Input: part model. Units: mm. Frame: model coordinates. Give positions to 0.01 mm unless a question says otherwise; leave off trailing zeros. Loops run counter-clockwise (first coordinate to the right, second up) from the corner with the lowest first, then second, coordinate; pieces in that order, holes last. Notation, with made-up numbers: M 12.5,71.25 L 45.5,71.25 A32 ccw 45.5,105.25 Z; hole C 13.25,24.25 d11. An arc over 180 degrees is marked long. Return JSON: item names as keys, results as strings. Group by question number.
```python
from build123d import *

# Parameters (mm, degrees)
F0_W         = 57.15
F0_H         = 69.85
F1_DEPTH     = 25.4
F2_R         = 3.556
F3_DEPTH     = 25.4
F4_T1_DEPTH  = 82.55
F5_T1_DEPTH  = 77.47
F5_T3_DEPTH  = 33.02
F5_T6_ANGLE  = 89.9999999979
F6_T1_DEPTH  = 64.77
F6_T3_DEPTH  = 33.02
F6_T6_ANGLE  = 89.9999999979
F7_T1_DEPTH  = 59.69
F7_T3_DEPTH  = 33.02
F7_T6_ANGLE  = 89.9999999979
F7_T8_ANGLE  = 89.9999999979
F8_T1_DEPTH  = 59.69
F8_T3_DEPTH  = 46.99
F8_T6_ANGLE  = 89.9999999979
F8_T8_ANGLE  = 90.0000000017
F8_T10_ANGLE = 90.0000000017
F8_T12_ANGLE = 89.9999999979


# Not quite as in the source:
# - a fillet or chamfer that OpenCascade refuses, or shapes differently, is made with other operations: its cross-section is extruded or revolved along the edge and cut away or added


with BuildPart() as f1:
    # F0 (on Top) → F1 (new body)
    with BuildSketch(Plane.XY):
        with Locations((-11.2585859209, 15.0406121326)):
            Rectangle(F0_W, F0_H)
    extrude(amount=F1_DEPTH)

    # F2 (on face) → F3 (cut)
    with BuildSketch(Plane.XY.offset(25.4)):
        with Locations((-30.9435859209, 42.3456121326)):
            Circle(F2_R)
        with Locations((8.4264140791, 42.3456121326)):
            Circle(F2_R)
        with Locations((-30.9435859209, -12.2643878674)):
            Circle(F2_R)
        with Locations((8.4264140791, -12.2643878674)):
            Circle(F2_R)
    extrude(amount=-F3_DEPTH, mode=Mode.SUBTRACT)

    # F4: fillet of radius 5.08 on 1 edges, made by hand

    # F4_s2 → F4_t1 (cut)
    with BuildSketch(Plane.YZ.offset(-52.5335859209)):
        with BuildLine():
            ThreePointArc((-14.8043878674, 25.4), (-18.3964903158, 23.9121024484), (-19.8843878674, 20.32))
            Line((-19.8843878674, 20.32), (-19.8843878674, 25.4))
            Line((-19.8843878674, 25.4), (-14.8043878674, 25.4))
        make_face()
    extrude(amount=F4_T1_DEPTH, mode=Mode.SUBTRACT)

    # F5: fillet of radius 5.08 on 1 edges, made by hand

    # F5_s2 → F5_t1 (cut)
    with BuildSketch(Plane.XZ.offset(-62.6656121326)):
        with BuildLine():
            ThreePointArc((17.3164140791, 20.32), (15.8285165275, 23.9121024484), (12.2364140791, 25.4))
            Line((12.2364140791, 25.4), (17.3164140791, 25.4))
            Line((17.3164140791, 25.4), (17.3164140791, 20.32))
        make_face()
    extrude(amount=F5_T1_DEPTH, mode=Mode.SUBTRACT)

    # F5_s4 → F5_t3 (cut)
    with BuildSketch(Plane.XY.offset(-12.7)):
        with BuildLine():
            ThreePointArc((17.3164140791, -14.8043878674), (15.8285165275, -18.3964903158), (12.2364140791, -19.8843878674))
            Line((12.2364140791, -19.8843878674), (17.3164140791, -19.8843878674))
            Line((17.3164140791, -19.8843878674), (17.3164140791, -14.8043878674))
        make_face()
    extrude(amount=F5_T3_DEPTH, mode=Mode.SUBTRACT)

    # F5_s5 → F5_t6 (revolve, cut)
    with BuildSketch(Plane.XY.offset(20.3199999999)):
        with BuildLine():
            ThreePointArc((17.3164140791, -14.8043878674), (15.8285165275, -18.3964903158), (12.2364140791, -19.8843878674))
            Line((12.2364140791, -19.8843878674), (17.3164140791, -19.8843878674))
            Line((17.3164140791, -19.8843878674), (17.3164140791, -14.8043878674))
        make_face()
    revolve(axis=Axis((17.3164140791, -14.8043878673, 20.3199999999), (-1, 0, 0)), revolution_arc=F5_T6_ANGLE, mode=Mode.SUBTRACT)

    # F6: fillet of radius 5.08 on 1 edges, made by hand

    # F6_s2 → F6_t1 (cut)
    with BuildSketch(Plane.YZ.offset(-52.5335859209)):
        with BuildLine():
            ThreePointArc((49.9656121326, 20.32), (48.477714581, 23.9121024484), (44.8856121326, 25.4))
            Line((44.8856121326, 25.4), (49.9656121326, 25.4))
            Line((49.9656121326, 25.4), (49.9656121326, 20.32))
        make_face()
    extrude(amount=F6_T1_DEPTH, mode=Mode.SUBTRACT)

    # F6_s4 → F6_t3 (cut)
    with BuildSketch(Plane.XY.offset(-12.7)):
        with BuildLine():
            ThreePointArc((12.2364140791, 49.9656121326), (15.8285165275, 48.477714581), (17.3164140791, 44.8856121326))
            Line((17.3164140791, 44.8856121326), (17.3164140791, 49.9656121326))
            Line((17.3164140791, 49.9656121326), (12.2364140791, 49.9656121326))
        make_face()
    extrude(amount=F6_T3_DEPTH, mode=Mode.SUBTRACT)

    # F6_s5 → F6_t6 (revolve, cut)
    with BuildSketch(Plane.YZ.offset(12.236414079)):
        with BuildLine():
            ThreePointArc((49.9656121326, 20.32), (48.477714581, 23.9121024484), (44.8856121326, 25.4))
            Line((44.8856121326, 25.4), (49.9656121326, 25.4))
            Line((49.9656121326, 25.4), (49.9656121326, 20.32))
        make_face()
    revolve(axis=Axis((12.236414079, 49.9656121326, 20.3199999999), (0, 1, 0)), revolution_arc=F6_T6_ANGLE, mode=Mode.SUBTRACT)

    # F7: fillet of radius 5.08 on 1 edges, made by hand

    # F7_s2 → F7_t1 (cut)
    with BuildSketch(Plane.XZ.offset(-44.8856121326)):
        with BuildLine():
            ThreePointArc((-39.8335859209, 20.32), (-38.3456883694, 23.9121024484), (-34.7535859209, 25.4))
            Line((-34.7535859209, 25.4), (-39.8335859209, 25.4))
            Line((-39.8335859209, 25.4), (-39.8335859209, 20.32))
        make_face()
    extrude(amount=F7_T1_DEPTH, mode=Mode.SUBTRACT)

    # F7_s4 → F7_t3 (cut)
    with BuildSketch(Plane.XY.offset(-12.7)):
        with BuildLine():
            ThreePointArc((-39.8335859209, -14.8043878674), (-38.3456883694, -18.3964903158), (-34.7535859209, -19.8843878674))
            Line((-34.7535859209, -19.8843878674), (-39.8335859209, -19.8843878674))
            Line((-39.8335859209, -19.8843878674), (-39.8335859209, -14.8043878674))
        make_face()
        with BuildLine():
            ThreePointArc((-34.7535859209, 49.9656121326), (-38.3456883694, 48.477714581), (-39.8335859209, 44.8856121326))
            Line((-39.8335859209, 44.8856121326), (-39.8335859209, 49.9656121326))
            Line((-39.8335859209, 49.9656121326), (-34.7535859209, 49.9656121326))
        make_face()
    extrude(amount=F7_T3_DEPTH, mode=Mode.SUBTRACT)

    # F7_s5 → F7_t6 (revolve, cut)
    with BuildSketch(Plane.XZ.offset(-44.8856121325)):
        with BuildLine():
            ThreePointArc((-39.8335859209, 20.32), (-38.3456883694, 23.9121024484), (-34.7535859209, 25.4))
            Line((-34.7535859209, 25.4), (-39.8335859209, 25.4))
            Line((-39.8335859209, 25.4), (-39.8335859209, 20.32))
        make_face()
    revolve(axis=Axis((-39.8335859209, 44.8856121325, 20.3199999999), (-1, 0, 0)), revolution_arc=F7_T6_ANGLE, mode=Mode.SUBTRACT)

    # F7_s7 → F7_t8 (revolve, cut)
    with BuildSketch(Plane.XY.offset(20.3199999999)):
        with BuildLine():
            ThreePointArc((-39.8335859209, -14.8043878674), (-38.3456883694, -18.3964903158), (-34.7535859209, -19.8843878674))
            Line((-34.7535859209, -19.8843878674), (-39.8335859209, -19.8843878674))
            Line((-39.8335859209, -19.8843878674), (-39.8335859209, -14.8043878674))
        make_face()
    revolve(axis=Axis((-39.8335859209, -14.8043878673, 20.3199999999), (-1, 0, 0)), revolution_arc=F7_T8_ANGLE, mode=Mode.SUBTRACT)

    # F8: fillet of radius 5.08 on 8 edges, made by hand

    # F8_s2 → F8_t1 (cut)
    with BuildSketch(Plane.XZ.offset(-44.8856121326)):
        with BuildLine():
            ThreePointArc((-34.7535859209, 0), (-38.3456883694, 1.4878975516), (-39.8335859209, 5.08))
            Line((-39.8335859209, 5.08), (-39.8335859209, 0))
            Line((-39.8335859209, 0), (-34.7535859209, 0))
        make_face()
        with BuildLine():
            ThreePointArc((12.2364140791, 0), (15.8285165275, 1.4878975516), (17.3164140791, 5.08))
            Line((17.3164140791, 5.08), (17.3164140791, 0))
            Line((17.3164140791, 0), (12.2364140791, 0))
        make_face()
    extrude(amount=F8_T1_DEPTH, mode=Mode.SUBTRACT)

    # F8_s4 → F8_t3 (cut)
    with BuildSketch(Plane.YZ.offset(-34.7535859209)):
        with BuildLine():
            ThreePointArc((49.9656121326, 5.08), (48.477714581, 1.4878975516), (44.8856121326, 0))
            Line((44.8856121326, 0), (49.9656121326, 0))
            Line((49.9656121326, 0), (49.9656121326, 5.08))
        make_face()
        with BuildLine():
            ThreePointArc((-14.8043878674, 0), (-18.3964903158, 1.4878975516), (-19.8843878674, 5.08))
            Line((-19.8843878674, 5.08), (-19.8843878674, 0))
            Line((-19.8843878674, 0), (-14.8043878674, 0))
        make_face()
    extrude(amount=F8_T3_DEPTH, mode=Mode.SUBTRACT)

    # F8_s5 → F8_t6 (revolve, cut)
    with BuildSketch(Plane.XZ.offset(14.8043878673)):
        with BuildLine():
            ThreePointArc((12.2364140791, 0), (15.8285165275, 1.4878975516), (17.3164140791, 5.08))
            Line((17.3164140791, 5.08), (17.3164140791, 0))
            Line((17.3164140791, 0), (12.2364140791, 0))
        make_face()
    revolve(axis=Axis((12.236414079, -14.8043878673, 0), (0, 0, -1)), revolution_arc=F8_T6_ANGLE, mode=Mode.SUBTRACT)

    # F8_s7 → F8_t8 (revolve, cut)
    with BuildSketch(Plane.YZ.offset(-34.753585921)):
        with BuildLine():
            ThreePointArc((-14.8043878674, 0), (-18.3964903158, 1.4878975516), (-19.8843878674, 5.08))
            Line((-19.8843878674, 5.08), (-19.8843878674, 0))
            Line((-19.8843878674, 0), (-14.8043878674, 0))
        make_face()
    revolve(axis=Axis((-34.753585921, -14.8043878675, 0), (0, 0, -1)), revolution_arc=F8_T8_ANGLE, mode=Mode.SUBTRACT)

    # F8_s9 → F8_t10 (revolve, cut)
    with BuildSketch(Plane.XZ.offset(-44.8856121327)):
        with BuildLine():
            ThreePointArc((-34.7535859209, 0), (-38.3456883693, 1.4878975516), (-39.8335859209, 5.08))
            Line((-39.8335859209, 5.08), (-39.8335859209, 0))
            Line((-39.8335859209, 0), (-34.7535859209, 0))
        make_face()
    revolve(axis=Axis((-34.753585921, 44.8856121327, 0), (0, 0, -1)), revolution_arc=F8_T10_ANGLE, mode=Mode.SUBTRACT)

    # F8_s11 → F8_t12 (revolve, cut)
    with BuildSketch(Plane.YZ.offset(12.236414079)):
        with BuildLine():
            ThreePointArc((44.8856121326, 0), (48.477714581, 1.4878975516), (49.9656121326, 5.08))
            Line((49.9656121326, 5.08), (49.9656121326, 0))
            Line((49.9656121326, 0), (44.8856121326, 0))
        make_face()
    revolve(axis=Axis((12.236414079, 44.8856121325, 0), (0, 0, -1)), revolution_arc=F8_T12_ANGLE, mode=Mode.SUBTRACT)


solid = f1.part
```
Item 1: Section C-C, the plane y = 19.5. Return loops of the section in (x, z), then the cut area to 3 significant figures.
Item 2: Section B-B, the plane x = 9. Return loops of the section in (y, z).
Item 3: Section D-D, the plane z = 3. Return loops of the section in (x, y).
Item 4: First-contact query: pin 1 Ø2 at (x, y) = (6, 19.5) entering from -Z; pin 2 Ø5.5 at (x, y) = (8.43, -12.26) entering from +Z. Flat tips, straight axial feed; report the tip coordinate or a pass-through.
Item 5: Material intervals for line 1 (X direction, y = 42, z = 12); line 2 (X direction, y = -11, z = 21); line 3 (Y direction, x = 9, z = 15.25), sorted ascending. Write a range as from..to.
Item 6: Section A-A, the plane z = 12.5. Return loops of the section in (x, y), then the cut area to 3 significant figures.
Item 7: Pull-direction query (Y, two-part tool) for faces 1 (the face through (17.316, 15, 13)), 2 (the face through (10.1, -15.4, 12.9)), 3 (the face through (-38.38, -18.36, 12.59)), 4 (the face through (-31.41, 45.87, 12.88)); classes: pulls with the +Y half, pulls with the -Y half, needs draft (parallel to the pull), parting line crosses it, or undercut.
Answer below:
{
 "1": {"outline": "M -39.83,5.08 A5.08 ccw -34.75,0 L 12.24,0 A5.08 ccw 17.32,5.08 L 17.32,20.32 A5.08 ccw 12.24,25.4 L -34.75,25.4 A5.08 ccw -39.83,20.32 Z", "area": "1,430 mm^2"},
 "2": {"outline": "M -19.88,5.08 A5.08 ccw -15.77,0.09 L -15.77,25.31 A5.08 ccw -19.88,20.32 Z; M -8.75,0 L 38.84,0 L 38.84,25.4 L -8.75,25.4 Z; M 45.86,0.09 A5.08 ccw 49.97,5.08 L 49.97,20.32 A5.08 ccw 45.86,25.31 Z"},
 "3": {"outline": "M -39.39,-14.8 A4.63 ccw -34.75,-19.44 L 12.24,-19.44 A4.63 ccw 16.87,-14.8 L 16.87,44.89 A4.63 ccw 12.24,49.52 L -34.75,49.52 A4.63 ccw -39.39,44.89 Z; hole C -30.94,-12.26 d7.11; hole C -30.94,42.35 d7.11; hole C 8.43,-12.26 d7.11; hole C 8.43,42.35 d7.11"},
 "4": {"pin 1": "z = 0", "pin 2": "through"},
 "5": {"line 1": "-39.83..-34.48, -27.4..4.89, 11.97..17.32", "line 2": "-39.79..-34.27, -27.62..5.1, 11.75..17.27", "line 3": "-19.88..-15.77, -8.75..38.84, 45.86..49.97"},
 "6": {"outline": "M -39.83,-14.8 A5.08 ccw -34.75,-19.88 L 12.24,-19.88 A5.08 ccw 17.32,-14.8 L 17.32,44.89 A5.08 ccw 12.24,49.97 L -34.75,49.97 A5.08 ccw -39.83,44.89 Z; hole C -30.94,-12.26 d7.11; hole C -30.94,42.35 d7.11; hole C 8.43,-12.26 d7.11; hole C 8.43,42.35 d7.11", "area": "3,810 mm^2"},
 "7": {"face 1": "needs draft", "face 2": "undercut", "face 3": "pulls with the -Y half", "face 4": "undercut"}
}
